Check sheet for the modelled part. Datum: model origin and axes. Units: mm. A direction names the side the tool comes from. Give positions to 0.01 mm unless a question says otherwise; leave off trailing zeros. Write each loop counter-clockwise with the first axis right and the second up, starting at its lowest first coordinate (ties: lowest second). Pieces come first, ordered by that corner, then holes. Notation, with made-up numbers: M 23.5,44.25 L 63.5,44.25 A33 ccw 63.5,75.25 Z; hole C 28,79.5 d4. An arc over 180 degrees is marked long. Use CSV: the item, a comma, the result in double quotes. Start each with the question number.
1. Scan lines: line 1 (X direction, y = -8.5, z = 11.75); line 2 (Y direction, x = 107.5, z = 10.5); line 3 (X direction, y = -16.5, z = 13.5). Record each from-to range of solid material in increasing order.
2. Cross-section at A-A, the plane x = -11.5. Enter the section's corners in (y, z) (3 decimals), and give its area (3 significant figures).
3. Access from +Z, -Z, +X, -X, +Y, -Y to the whole of each face (thin tool, end or side, straight path). Record for faces 5 (the face through (0, -10, 0)), 6 (the face through (0, -10, 3.175)), 7 (the face through (-131.21, -6.942, 6.953)).
4. Depth check by flat-ended pin: P1, Ø6, axis at y = -1.5, z = 9.5, coming from the -X side. Enter the tip coordinate at first touch or a pass-through.
5. Mould release check, pull along X, two halves, no side actions. Record for faces 1 (the face through (0, 2.099, 9)), 2 (the face through (-128.079, -10.1, 13.3)), 3 (the face through (127.826, -10, 11)), 4 (the face through (131.001, -10, 9)): +X half, -X half, draft (parallel to the pull), parting line (faces both ways), or undercut.
6. Cross-section at B-B, the plane y = -9. Enter the section's corners in (x, z) (3 decimals), and give its area (3 significant figures).
from build123d import *

# Parameters (mm, degrees)
F0_W     = 252.73
F0_H     = 17.78
F1_DEPTH = 3.175
F0_W_2   = 259.08
F0_H_2   = 24.13
F2_DEPTH = 18.542
F3_R     = 3.81
F4_DEPTH = 6.35


with BuildPart() as f1:
    # F0 (on Top) → F1 (new body)
    with BuildSketch(Plane.XY):
        with Locations((1.460627, -9.965609)):
            Rectangle(F0_W, F0_H)
    extrude(amount=F1_DEPTH)

    # F0 (on Top) → F2 (join)
    with BuildSketch(Plane.XY):
        with Locations((1.460627, -9.965609)):
            Rectangle(F0_W_2, F0_H_2)
        with Locations((1.460627, -9.965609)):
            Rectangle(F0_W, F0_H, mode=Mode.SUBTRACT)
    extrude(amount=F2_DEPTH)

    # F3 (on face) → F4 (join)
    with BuildSketch(Plane(origin=(-128.079373, 0, 0), x_dir=(0, -1, 0), z_dir=(-1, 0, 0))):
        with Locations((9.965609, 9.271)):
            Circle(F3_R)
    extrude(amount=F4_DEPTH)


solid = f1.part
Worked answers:
1,line 1,"x = -134.43 to -124.9, 127.83 to 131"
1,line 2,"y = -22.03 to -18.86, -1.08 to 2.1"
1,line 3,"x = -128.08 to -124.9, 127.83 to 131"
2,outline,"M -22.031,0 L 2.099,0 L 2.099,18.542 L -1.076,18.542 L -1.076,3.175 L -18.856,3.175 L -18.856,18.542 L -22.031,18.542 Z"
2,area,"174 mm^2"
3,face 5,"-Z, +X, -X, +Y, -Y"
3,face 6,"+Z"
3,face 7,"-X"
4,P1,"stops at x = -128.08"
5,face 1,"draft"
5,face 2,"-X half"
5,face 3,"undercut"
5,face 4,"+X half"
6,outline,"M -134.429,5.585 L -128.079,5.585 L -128.079,0 L 131.001,0 L 131.001,18.542 L 127.826,18.542 L 127.826,3.175 L -124.904,3.175 L -124.904,18.542 L -128.079,18.542 L -128.079,12.957 L -134.429,12.957 Z"
6,area,"967 mm^2"
